from build123d import *

# Parameters (mm, degrees)
F0_W     = 50
F0_H     = 50
F0_R     = 1.05
F1_DEPTH = 3
F2_W     = 15
F2_H     = 12.085
F3_DEPTH = 3.001
F4_R     = 2.04
F5_DEPTH = 3.001
F7_DEPTH = 3.001
F8_W     = 8.9
F8_H     = 8.9
F9_DEPTH = 3.001
F10_R    = 5.08
F11_R    = 2.54
F12_R    = 2.54


with BuildPart() as f1:
    # F0 (on Front) → F1 (new body)
    with BuildSketch(Plane.XZ):
        with Locations((25, 25)):
            Rectangle(F0_W, F0_H)
        with Locations((7.11, 27.33)):
            Circle(F0_R, mode=Mode.SUBTRACT)
        with Locations((7.11, 45)):
            Circle(F0_R, mode=Mode.SUBTRACT)
        with Locations((42.89, 27.33)):
            Circle(F0_R, mode=Mode.SUBTRACT)
        with Locations((42.89, 45)):
            Circle(F0_R, mode=Mode.SUBTRACT)
    extrude(amount=F1_DEPTH)

    # F2 (on face) → F3 (cut, through all)
    with BuildSketch(Plane.XZ.offset(3)):
        with Locations((7.5, 36.5725)):
            Rectangle(F2_W, F2_H)
    extrude(amount=-F3_DEPTH, mode=Mode.SUBTRACT)

    # F4 (on face) → F5 (cut, through all)
    with BuildSketch(Plane.XZ.offset(3)):
        with Locations((8.4, 8.9)):
            Circle(F4_R)
        with Locations((41.6, 8.9)):
            Circle(F4_R)
    extrude(amount=-F5_DEPTH, mode=Mode.SUBTRACT)

    # F6 (on face) → F7 (cut, through all)
    with BuildSketch(Plane.XZ.offset(3)):
        Polygon((37.3, 29.38), (46.19, 29.38), (46.19, 0), (50, 0), (50, 29.38), (50, 42.95), (50, 50), (46.19, 50), (46.19, 42.95), (37.3, 42.95), align=None)
    extrude(amount=-F7_DEPTH, mode=Mode.SUBTRACT)

    # F8 (on face) → F9 (cut, through all)
    with BuildSketch(Plane(origin=(0, 0, 0), x_dir=(-1, 0, 0), z_dir=(0, 1, 0))):
        with Locations((-15, 42.615)):
            Rectangle(F8_W, F8_H)
    extrude(amount=-F9_DEPTH, mode=Mode.SUBTRACT)

    # F10
    f10_edges = [f1.edges().sort_by_distance(p)[0] for p in [
        (0, -1.5, 50),
        (0, -1.5, 0),
    ]]
    fillet(f10_edges, radius=F10_R)

    # F11
    f11_edges = [f1.edges().sort_by_distance(p)[0] for p in [
        (19.45, -1.5, 47.065),
        (19.45, -1.5, 38.165),
        (10.55, -1.5, 47.065),
    ]]
    fillet(f11_edges, radius=F11_R)

    # F12
    f12_edges = [f1.edges().sort_by_distance(p)[0] for p in [
        (46.19, -1.5, 50),
        (46.19, -1.5, 29.38),
        (46.19, -1.5, 42.95),
        (0, -1.5, 42.615),
        (0, -1.5, 30.53),
        (46.19, -1.5, 0),
    ]]
    fillet(f12_edges, radius=F12_R)


solid = f1.part
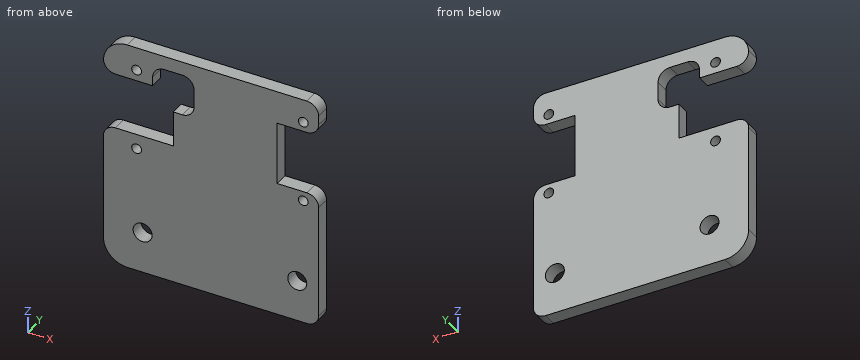
The model under review builds one solid part; all positions refer to its coordinate system, in mm. Coordinates: 2 decimals unless noted, no trailing zeros. Write each loop counter-clockwise with the first axis right and the second up, starting at its lowest first coordinate (ties: lowest second). Pieces come first, ordered by that corner, then holes. Notation, with made-up numbers: (43, -8.75) - (94, -8.75) arc R21 ccw to (94, 17.25) - close; hole circle Ø2 at (-19, -14). An arc over 180 degrees is marked (long way). Answer as CSV lines item,"result".
(1) We need section C-C (x = 12). Give the boundary of the cut face in (y, z), plus the area to 3 significant figures.
Data:
outline,"(-3, 0) - (0, 0) - (0, 30.53) - (-3, 30.53) - close; (-3, 46.82) - (0, 46.82) - (0, 50) - (-3, 50) - close"
area,"101 mm2"
(2) For line 1 along Z through (x, y) = (41.6, -1.15); line 2 along Z through (x, y) = (7.5, -1.25) (3 decimals); line 3 along X through (y, z) = (-1.45, 27), list the stretches that pass through material, from the lowest coordinate up. Write a range as [from, to].
Data:
line 1,"z = [0, 6.86], [10.94, 29.38], [42.95, 50]"
line 2,"z = [0, 7.069], [10.731, 26.355], [28.305, 30.53], [42.615, 44.025], [45.975, 50]"
line 3,"x = [0, 6.11], [8.11, 41.89], [43.89, 46.18]"
(3) We need section D-D (y = -1.1). Count the separate pieces of the cut face and the enclosed holes in it, plus the area to 3 significant figures.
Data:
separate pieces,"1"
enclosed holes,"6"
area,"1,890 mm2"
(4) We need section A-A (z = 8.9). Give the boundary of the cut face in (x, y), plus the area to 3 significant figures.
Data:
outline,"(0, -3) - (6.36, -3) - (6.36, 0) - (0, 0) - close; (10.44, -3) - (39.56, -3) - (39.56, 0) - (10.44, 0) - close; (43.64, -3) - (46.19, -3) - (46.19, 0) - (43.64, 0) - close"
area,"114 mm2"
(5) We need section B-B (x = 42.89). Give the boundary of the cut face in (y, z), plus the area to 3 significant figures.
Data:
outline,"(-3, 0) - (0, 0) - (0, 7.32) - (-3, 7.32) - close; (-3, 10.48) - (0, 10.48) - (0, 26.28) - (-3, 26.28) - close; (-3, 28.38) - (0, 28.38) - (0, 29.38) - (-3, 29.38) - close; (-3, 42.95) - (0, 42.95) - (0, 43.95) - (-3, 43.95) - close; (-3, 46.05) - (0, 46.05) - (0, 50) - (-3, 50) - close"
area,"87.2 mm2"
(6) Clearance check with flat-ended pins moving along their axes: pin 1 Ø1 at (y, z) = (-1, 38.5) entering from -X; pin 2 Ø3.5 at (x, z) = (7.11, 45) entering from +Y; pin 3 Ø3.5 at (x, z) = (8.4, 8.9) entering from +Y; pin 4 Ø0.9 at (y, z) = (-1, 38) entering from +X. State where each tip first meets the part, or that it passes through.
Data:
pin 1,"stops at x = 15"
pin 2,"stops at y = 0"
pin 3,"passes through"
pin 4,"stops at x = 37.3"
